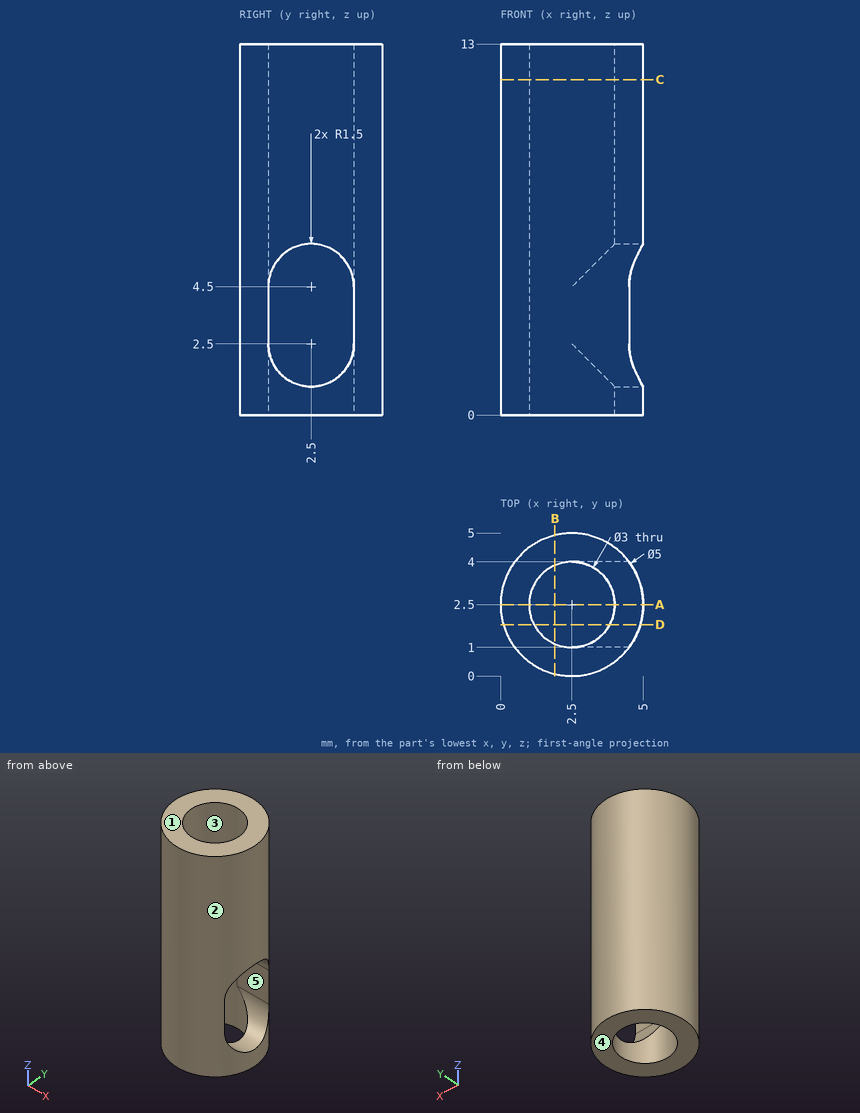
Geometry: see drawing. Coordinates: mm, zero at the bounding-box minimum. A direction names the side the tool comes from. Give positions to 0.01 mm unless a question says otherwise; leave off trailing zeros. Order: outer loops, then holes, each group sorted by start corner. A loop starts at its lowest first (then second) coordinate and runs counter-clockwise, first axis right, second up. Notation, with made-up numbers: M 28,57.5 L 71,57.5 A23 ccw 71,71.5 Z; hole C 65.5,36 d2. An arc over 180 degrees is marked long. Answer as CSV lines item,"result". Start each with the question number.
1) Line query: line 1 (Y direction, x = 2.55, z = 11.75); line 2 (Z direction, x = 4.2, y = 2.6); line 3 (Y direction, x = 3, z = 8). Output: solid intervals per line, ascending. Write a range as from..to.
2) First-contact query: P1, Ø1, axis at x = 3, z = 9, coming from the -Y side; P2, Ø1.5, axis at y = 1.5, z = 3, coming from the +X side; P3, Ø2, axis at y = 4, z = 10, coming from the +X side. Flat tips, straight axial feed; report the tip coordinate or a pass-through.
3) Cut plane C-C (z = 11.75). Output: boundary loops of the cut face in (x, y), then the cut area to 3 significant figures.
4) Set-up query: the marked faces 4 and 5. Return all of +Z, -Z, +X, -X, +Y, -Y with unobstructed straight access to the full face (end or side cutting, diameter ignored); none if empty.
5) Cut plane A-A (y = 2.5). Output: boundary loops of the cut face in (x, z).
6) Mould query, pull axis X, two halves, no side actions, for the marked faces 1, 2 and 3. Classes: +X half, -X half, draft (parallel to the pull), parting line (faces both ways), or undercut.
7) Cut plane D-D (y = 1.8). Output: boundary loops of the cut face in (x, z), then the cut area to 3 significant figures.
8) Cut plane B-B (x = 1.9). Output: boundary loops of the cut face in (y, z).
Findings below:
1,line 1,"y = 0..1, 4..5"
1,line 2,"z = 0..1, 6..13"
1,line 3,"y = 0.05..1.09, 3.91..4.95"
2,P1,"stops at y = 0"
2,P2,"stops at x = 4.5"
2,P3,"stops at x = 4.95"
3,outline,"C 2.5,2.5 d5; hole C 2.5,2.5 d3"
3,area,"12.6 mm²"
4,face 4,"-Z, +X, -X, +Y, -Y"
4,face 5,"+X"
5,outline,"M 0,0 L 1,0 L 1,13 L 0,13 Z; M 4,0 L 5,0 L 5,1 L 4,1 Z; M 4,6 L 5,6 L 5,13 L 4,13 Z"
6,face 1,"draft"
6,face 2,"parting line"
6,face 3,"undercut"
7,outline,"M 0.1,0 L 1.17,0 L 1.17,13 L 0.1,13 Z; M 3.83,0 L 4.9,0 L 4.9,1.17 L 3.83,1.17 Z; M 3.83,5.83 L 4.9,5.83 L 4.9,13 L 3.83,13 Z"
7,area,"22.9 mm²"
8,outline,"M 0.07,0 L 1.13,0 L 1.13,13 L 0.07,13 Z; M 3.87,0 L 4.93,0 L 4.93,13 L 3.87,13 Z"
